The drawing under review shows one solid part. Ordinate dimensions are in mm from its lowest x, y, z. A direction names the side the tool comes from. Coordinates: 2 decimals unless noted, no trailing zeros. Order: outer loops, then holes, each group sorted by start corner. A loop starts at its lowest first (then second) coordinate and runs counter-clockwise, first axis right, second up. Notation, with made-up numbers: M -32,17 L 8,17 A26 ccw 8,50 Z; hole C 68,-9 d2. An arc over 180 degrees is marked long. Answer as a JSON object with one key per item and string values.
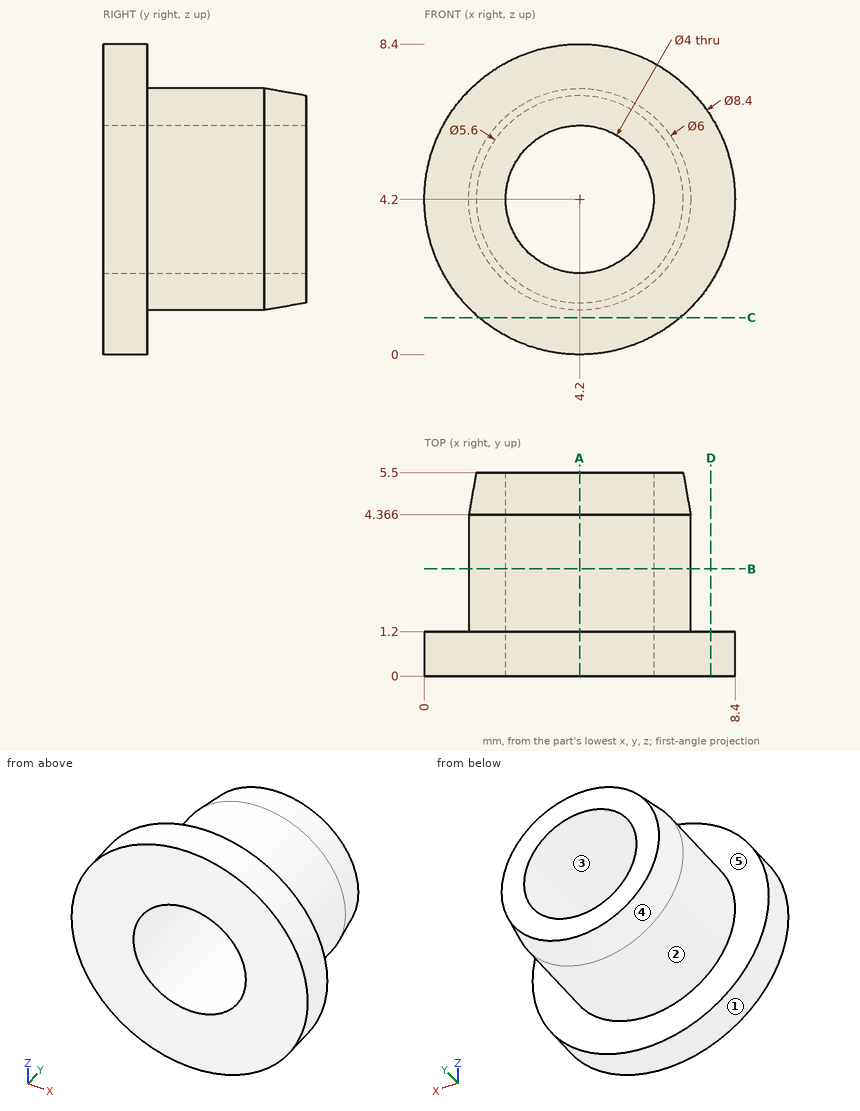
1) To check wall thickness, follow L1, parallel to Z at x = 4.2, y = 1.8; L2, parallel to Y at x = 1.5, z = 6. State the ranges of each line that lie inside material, in increasing order.
Taken from the geometry:
{"L1": "z = 1.2 to 2.2, 6.2 to 7.2", "L2": "y = 0 to 1.2"}
2) Add section B-B (y = 2.9). State the section outline as (x, z) points, and give its area (3 significant figures).
Taken from the geometry:
{"outline": "C 4.2,4.2 d6; hole C 4.2,4.2 d4", "area": "15.7 mm2"}
3) Insertion check: pin 1 Ø1 at (y, z) = (3.5, 5) entering from -X (3 decimals); pin 2 Ø1 at (x, z) = (5, 3.5) entering from +Y; pin 3 Ø2 at (x, y) = (4, 4) entering from +Z. Each pin has a flat end and moves straight along its axis. Give the tip position at first contact, or say it passes through.
Taken from the geometry:
{"pin 1": "stops at x = 1.215", "pin 2": "passes through", "pin 3": "stops at z = 7.2"}
4) Add section D-D (x = 7.75). State the section outline as (y, z) points.
Taken from the geometry:
{"outline": "M 0,1.96 L 1.2,1.96 L 1.2,6.44 L 0,6.44 Z"}
5) Add section C-C (z = 1). State the section outline as (x, y) points.
Taken from the geometry:
{"outline": "M 1.48,0 L 6.92,0 L 6.92,1.2 L 1.48,1.2 Z"}
6) Mouldability with a two-part tool opening along Z and no side actions: class the marked faces 3, 4 and 5 as released by +Z, released by -Z, zero draft, split by the parting line, or undercut.
Taken from the geometry:
{"face 3": "undercut", "face 4": "split by the parting line", "face 5": "zero draft"}
7) Add section A-A (x = 4.2). State the section outline as (y, z) points.
Taken from the geometry:
{"outline": "M 0,0 L 1.2,0 L 1.2,1.2 L 4.37,1.2 L 5.5,1.4 L 5.5,2.2 L 0,2.2 Z; M 0,6.2 L 5.5,6.2 L 5.5,7 L 4.37,7.2 L 1.2,7.2 L 1.2,8.4 L 0,8.4 Z"}
8) Tool access review of the marked faces 1 and 2: name each direction out of +Z, -Z, +X, -X, +Y, -Y from which nothing blocks a thin tool from reaching the whole face with its end or side.
Taken from the geometry:
{"face 1": "+Y, -Y", "face 2": "+Y"}
